Here's the drawing with two shaded views (mm, measured from the low corner). I have some questions. A direction names the side the tool comes from. Round coordinates to 2 decimals unless told otherwise and drop trailing zeros. Loops run counter-clockwise (first coordinate to the right, second up) from the corner with the lowest first, then second, coordinate; pieces in that order, holes last. Notation, with made-up numbers: M 35.25,26 L 43.25,26 A30 cw 43.25,55 Z; hole C 15,-4.75 d6. An arc over 180 degrees is marked long. Write each question's results on one line, items separated by ' | '. Start each with the question number.
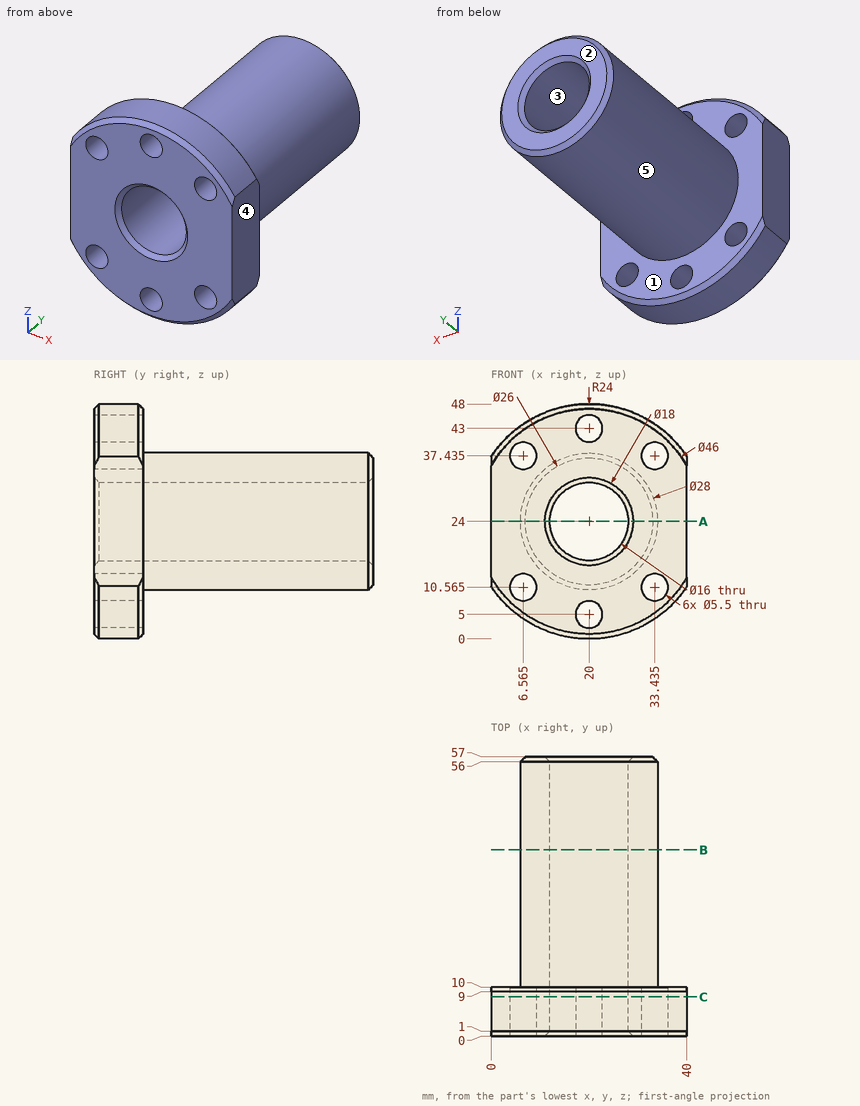
Item 1: If we section it at B-B on y = 38: Please give me the cut outline in (x, z).
Item 2: Which directions (+Z, -Z, +X, -X, +Y, -Y) give clear straight access to the entire face, cutting with the end or side of a thin tool? Please do the marked faces 1 and 2.
Item 3: If we section it at A-A on z = 24: Please give me the cut outline in (x, y).
Item 4: I'm going to push flat-ended pins straight in: pin 1 (4 mm diameter, centred on x = 24, y = 32.5, fed in from -Z); pin 2 (8 mm diameter, centred on x = 15, y = 46.5, fed in from -Z); pin 3 (9 mm diameter, centred on x = 33.44, z = 10.56, fed in from +Y). Where does each tip first touch, or does it pass through?
Item 5: I need wall thicknesses on L1, parallel to X at y = 19, z = 24; L2, parallel to X at y = 3, z = 11.5; L3, parallel to Z at x = 20.5, y = 27. Which ranges of each line are inside material? Lowest first, please.
Item 6: If we mould it in two halves opening along Z, with no side actions, what happens to the marked faces 3, 4 and 5? For each: released by +Z, released by -Z, zero draft, split by the parting line, or undercut.
Item 7: If we section it at C-C on y = 8: Count the separate pieces of the cut face and the enclosed holes in it, and give its area (3 significant figures).
Numbers:
1) outline: C 20,24 d28; hole C 20,24 d16
2) face 1: +Y | face 2: +Z, -Z, +X, -X, +Y
3) outline: M 0,0 L 11,0 L 12,1 L 12,56 L 11,57 L 7,57 L 6,56 L 6,10 L 0,10 Z; M 28,1 L 29,0 L 40,0 L 40,10 L 34,10 L 34,56 L 33,57 L 29,57 L 28,56 Z
4) pin 1: z = 10.14 | pin 2: z = 10.04 | pin 3: y = 10
5) L1: 6 to 12, 28 to 34 | L2: 0 to 3.98, 9.15 to 30.85, 36.02 to 40 | L3: 10.01 to 16.02, 31.98 to 37.99
6) face 3: undercut | face 4: zero draft | face 5: split by the parting line
7) separate pieces: 1 | enclosed holes: 7 | area: 1,320 mm²
